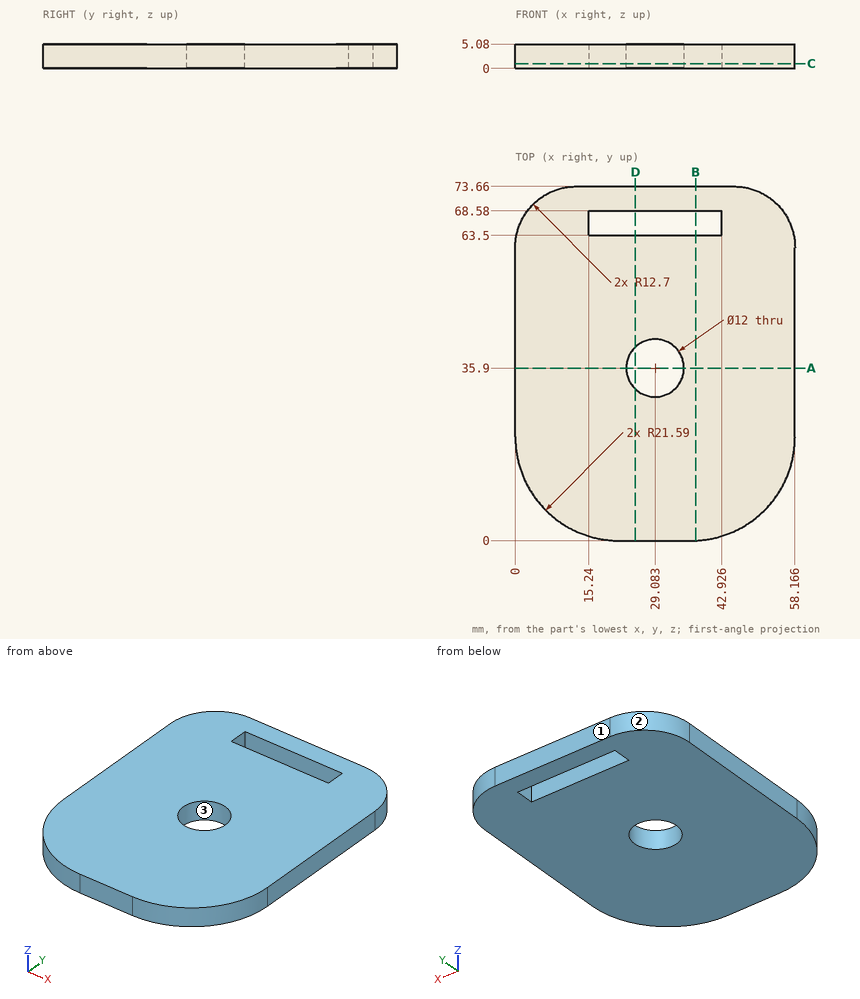
The figure shows three views and two pictorial views of one solid part (mm, origin at its lowest corner). Answer the questions. Coordinates: 2 decimals unless noted, no trailing zeros. Loops run counter-clockwise (first coordinate to the right, second up) from the corner with the lowest first, then second, coordinate; pieces in that order, holes last. Notation, with made-up numbers: (47, 63) - (71, 63) arc R33 ccw to (71, 97) - close; hole circle Ø8 at (-21.75, 45.5). An arc over 180 degrees is marked (long way). Use a Markdown table: item, result. Add a question column.
1) The part is cut by section C-C, the plane z = 1. Give the vertices of the cut face in (x, y).
2) Given pin 1 (1.5 mm diameter, centred on y = 65.5, z = 3, fed in from +X), flat-ended and moving along its own axis, determine where the tip first touches the part or whether it passes through.
3) Find the intervals of material crossed by line 1 (Y direction, x = 26, z = 2.95); line 2 (Y direction, x = 18, z = 4.7); line 3 (Y direction, x = 30.5, z = 2.7), in increasing order.
4) The mould has two halves that part along X. Classify the marked faces 1, 2 and 3: released by +X, released by -X, zero draft, split by the parting line, or undercut.
5) The part is cut by section A-A, the plane y = 35.9. Give the vertices of the cut face in (x, z), and give its area (3 significant figures).
6) The part is cut by section D-D, the plane x = 25. Give the vertices of the cut face in (y, z).
7) The part is cut by section B-B, the plane x = 37.5. Give the vertices of the cut face in (y, z).
Here are the results:
| question | item | result |
|---|---|---|
| 1 | outline | (0, 21.59) arc R21.59 ccw to (21.59, 0) - (36.58, 0) arc R21.59 ccw to (58.17, 21.59) - (58.17, 60.96) arc R12.7 ccw to (45.47, 73.66) - (12.7, 73.66) arc R12.7 ccw to (0, 60.96) - close; hole (15.24, 63.5) - (42.93, 63.5) - (42.93, 68.58) - (15.24, 68.58) - close; hole circle Ø12 at (29.08, 35.9) |
| 2 | pin 1 | stops at x = 57.59 |
| 3 | line 1 | y = 0 to 30.75, 41.05 to 63.5, 68.58 to 73.66 |
| 3 | line 2 | y = 0.3 to 63.5, 68.58 to 73.66 |
| 3 | line 3 | y = 0 to 30.07, 41.73 to 63.5, 68.58 to 73.66 |
| 4 | face 1 | zero draft |
| 4 | face 2 | released by -X |
| 4 | face 3 | undercut |
| 5 | outline | (0, 0) - (23.08, 0) - (23.08, 5.08) - (0, 5.08) - close; (35.08, 0) - (58.17, 0) - (58.17, 5.08) - (35.08, 5.08) - close |
| 5 | area | 235 mm^2 |
| 6 | outline | (0, 0) - (31.5, 0) - (31.5, 5.08) - (0, 5.08) - close; (40.3, 0) - (63.5, 0) - (63.5, 5.08) - (40.3, 5.08) - close; (68.58, 0) - (73.66, 0) - (73.66, 5.08) - (68.58, 5.08) - close |
| 7 | outline | (0.02, 0) - (63.5, 0) - (63.5, 5.08) - (0.02, 5.08) - close; (68.58, 0) - (73.66, 0) - (73.66, 5.08) - (68.58, 5.08) - close |
